```python
from build123d import *

# Parameters (mm, degrees)
BOSS_EXTRUDE1_DEPTH = 3
SKETCH2_W           = 4
SKETCH2_H           = 5
BOSS_EXTRUDE2_DEPTH = 5
SKETCH3_R           = 1.75
CUT_EXTRUDE1_DEPTH  = 14
FILLET1_R           = 1
SKETCH5_R           = 2
CUT_EXTRUDE2_DEPTH  = 5
SKETCH7_R           = 2
CUT_EXTRUDE3_DEPTH  = 5
FILLET2_R           = 1


with BuildPart() as part:
    # Sketch1 → Boss-Extrude1 (new body)
    with BuildSketch(Plane.XY):
        Polygon((17.84234206, -3.321281539), (17.84234206, -10.791281539), (17.84234206, -11.641281539), (16.99234206, -11.641281539), (-15.30765794, -11.641281539), (-16.98765794, -11.641281539), (-16.98765794, -9.505481629), (-16.98765794, -2.491281539), (-16.98765794, -1.641281539), (-16.13765794, -1.641281539), (16.16234206, -1.641281539), (17.84234206, -1.641281539), align=None)
    extrude(amount=BOSS_EXTRUDE1_DEPTH)

    # Sketch2 → Boss-Extrude2 (add)
    with BuildSketch(Plane.XY.offset(3)):
        with Locations((-4.554565942, -5.902432564)):
            Rectangle(SKETCH2_W, SKETCH2_H)
        with Locations((3.578766058, -5.902432564)):
            Rectangle(SKETCH2_W, SKETCH2_H)
    extrude(amount=BOSS_EXTRUDE2_DEPTH)

    # Sketch3 → Cut-Extrude1 (cut)
    with BuildSketch(Plane(origin=(5.578766058, 0, 0), x_dir=(0, 0, -1), z_dir=(1, 0, 0))):
        with Locations(Location((-5.5, -5.902432564, 0), (0, 0, 90))):
            Circle(SKETCH3_R)
    extrude(amount=-CUT_EXTRUDE1_DEPTH, mode=Mode.SUBTRACT)

    # Fillet1
    fillet1_edges = [part.edges().sort_by_distance(p)[0] for p in [
        (-16.98765794, -11.641281539, 1.5),
        (-16.98765794, -1.641281539, 1.5),
        (17.84234206, -1.641281539, 1.5),
        (17.84234206, -11.641281539, 1.5),
    ]]
    fillet(fillet1_edges, radius=FILLET1_R)

    # Sketch5 → Cut-Extrude2 (cut)
    with BuildSketch(Plane.XY.offset(3)):
        with Locations((-12.48765794, -6.641281539)):
            Circle(SKETCH5_R)
    extrude(amount=-CUT_EXTRUDE2_DEPTH, mode=Mode.SUBTRACT)

    # Sketch7 → Cut-Extrude3 (cut)
    with BuildSketch(Plane.XY.offset(3)):
        with Locations((13.34234206, -6.641281539)):
            Circle(SKETCH7_R)
    extrude(amount=-CUT_EXTRUDE3_DEPTH, mode=Mode.SUBTRACT)

    # Fillet2
    fillet2_edges = [part.edges().sort_by_distance(p)[0] for p in [
        (-4.554565942, -8.402432564, 8),
        (-4.554565942, -3.402432564, 8),
        (3.578766058, -3.402432564, 8),
        (3.578766058, -8.402432564, 8),
    ]]
    fillet(fillet2_edges, radius=FILLET2_R)


solid = part.part
```
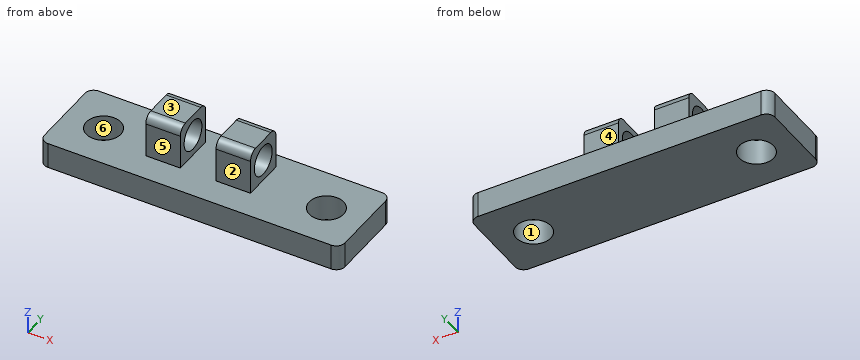
Read the model definition and answer for the solid it produces. Units are mm, in the model's axes. Face numbers are marked on the shaded views. A direction names the side the tool comes from. Coordinates: 2 decimals unless noted, no trailing zeros. Order: outer loops, then holes, each group sorted by start corner. A loop starts at its lowest first (then second) coordinate and runs counter-clockwise, first axis right, second up. Notation, with made-up numbers: (24, 65.25) - (33, 65.25) arc R20 ccw to (33, 100.25) - close; hole circle Ø3 at (18, 59). An arc over 180 degrees is marked (long way). Answer as a JSON object with one key per item and string values. Group by question number.
Item 1: The mould has two halves that part along Y. Classify the marked faces 1, 2 and 3: +Y half, -Y half, draft (parallel to the pull), parting line (faces both ways), or undercut.
Item 2: Flat-ended cylindrical pins translate along their axes: P1, Ø2, axis at x = 1.5, y = -7, coming from the +Z side; P2, Ø3, axis at x = -12.49, y = -6.64, coming from the +Z side; P3, Ø4, axis at y = -5.9, z = 5.5, coming from the -X side; P4, Ø2.5, axis at y = -6.5, z = 4.5, coming from the +X side. Find the tip coordinate at first contact, or state that the pin passes through.
Item 3: Section A-A (z = 5.5) is taken. Give the vertices of the cut face in (x, y), plus the area to 3 significant figures.
Item 4: Section C-C (y = -5.25) is taken. Give the vertices of the cut face in (x, z), plus the area to 3 significant figures.
Item 5: A tool of negligible diameter and unlimited length cuts with its end or side. For the marked faces 4, 5 and 6, from which of +Z, -Z, +X, -X, +Y, -Y can it reach the whole face along a straight path? Write none if from no direction.
Item 6: Consider probe 1 along X at (y, z) = (-8.25, 4.75); probe 2 along Z at (x, y) = (-11, -4.5). Determine where each line is inside the solid, lowest interval first. Write a range as from..to.
Item 7: Section B-B (x = 5) is taken. Give the vertices of the cut face in (y, z), plus the area to 3 significant figures.
Results are:
{
 "1": {"face 1": "undercut", "face 2": "-Y half", "face 3": "draft"},
 "2": {"P1": "stops at z = 8", "P2": "passes through", "P3": "stops at x = -6.55", "P4": "stops at x = 5.58"},
 "3": {"outline": "(-6.55, -8.4) - (-2.55, -8.4) - (-2.55, -7.65) - (-6.55, -7.65) - close; (-6.55, -4.15) - (-2.55, -4.15) - (-2.55, -3.4) - (-6.55, -3.4) - close; (1.58, -8.4) - (5.58, -8.4) - (5.58, -7.65) - (1.58, -7.65) - close; (1.58, -4.15) - (5.58, -4.15) - (5.58, -3.4) - (1.58, -3.4) - close", "area": "12.0 mm^2"},
 "4": {"outline": "(-16.99, 0) - (-13.92, 0) - (-13.92, 3) - (-16.99, 3) - close; (-11.05, 0) - (11.91, 0) - (11.91, 3) - (5.58, 3) - (5.58, 3.88) - (1.58, 3.88) - (1.58, 3) - (-2.55, 3) - (-2.55, 3.88) - (-6.55, 3.88) - (-6.55, 3) - (-11.05, 3) - close; (-6.55, 7.12) - (-2.55, 7.12) - (-2.55, 8) - (-6.55, 8) - close; (1.58, 7.12) - (5.58, 7.12) - (5.58, 8) - (1.58, 8) - close; (14.78, 0) - (17.84, 0) - (17.84, 3) - (14.78, 3) - close", "area": "101 mm^2"},
 "5": {"face 4": "+Z, +X, -X, +Y", "face 5": "+Z, +X, -X, -Y", "face 6": "+Z, -Z"},
 "6": {"probe 1": "x = -6.55..-2.55, 1.58..5.58", "probe 2": "z = 0..3"},
 "7": {"outline": "(-11.64, 0) - (-1.64, 0) - (-1.64, 3) - (-3.4, 3) - (-3.4, 7) arc R1 ccw to (-4.4, 8) - (-7.4, 8) arc R1 ccw to (-8.4, 7) - (-8.4, 3) - (-11.64, 3) - close; hole circle Ø3.5 at (-5.9, 5.5)", "area": "44.9 mm^2"}
}
